```python
from build123d import *

# Parameters (mm, degrees)
SKETCH_W          = 28
SKETCH_H          = 22
PAD_DEPTH         = 52
FILLET_R          = 2
FILLET001_R       = 2
FILLET002_R       = 2
FILLET003_R       = 2
BOX_W             = 48
BOX_H             = 22.4
BOX_DEPTH         = 5.7
CYLINDER_R        = 1.5
CYLINDER_DEPTH    = 6
CYLINDER001_R     = 1.5
CYLINDER001_DEPTH = 6


with BuildPart() as part:
    # Sketch → Pad (new body)
    with BuildSketch(Plane.XZ):
        Rectangle(SKETCH_W, SKETCH_H)
    extrude(amount=PAD_DEPTH)

    # Fillet
    fillet_edges = [part.edges().sort_by_distance(p)[0] for p in [
        (-14, -26, 11),
    ]]
    fillet(fillet_edges, radius=FILLET_R)

    # Fillet001
    fillet001_edges = [part.edges().sort_by_distance(p)[0] for p in [
        (-14, -26, -11),
    ]]
    fillet(fillet001_edges, radius=FILLET001_R)

    # Fillet002
    fillet002_edges = [part.edges().sort_by_distance(p)[0] for p in [
        (14, -26, 11),
    ]]
    fillet(fillet002_edges, radius=FILLET002_R)

    # Fillet003
    fillet003_edges = [part.edges().sort_by_distance(p)[0] for p in [
        (14, -26, -11),
    ]]
    fillet(fillet003_edges, radius=FILLET003_R)

    # Box → Box (join)
    with BuildSketch(Plane(origin=(-24, 5.7, -11.2), x_dir=(1, 0, 0), z_dir=(0, -1, 0))):
        with Locations((24, 11.2)):
            Rectangle(BOX_W, BOX_H)
    extrude(amount=BOX_DEPTH)

    # Cylinder → Cylinder (join)
    with BuildSketch(Plane(origin=(-20, 0, 0), x_dir=(1, 0, 0), z_dir=(0, -1, 0))):
        Circle(CYLINDER_R)
    extrude(amount=CYLINDER_DEPTH)

    # Cylinder001 → Cylinder001 (join)
    with BuildSketch(Plane(origin=(20, 0, 0), x_dir=(1, 0, 0), z_dir=(0, -1, 0))):
        Circle(CYLINDER001_R)
    extrude(amount=CYLINDER001_DEPTH)


solid = part.part
```
Model file for the job. Use its own axes, mm. A direction names the side the tool comes from. Coordinates: 2 decimals unless noted, no trailing zeros. Loops run counter-clockwise (first coordinate to the right, second up) from the corner with the lowest first, then second, coordinate; pieces in that order, holes last. Notation, with made-up numbers: (26, 61.25) - (45, 61.25) arc R22 ccw to (45, 76.25) - close; hole circle Ø9 at (53, 41.25). An arc over 180 degrees is marked (long way). Answer as a JSON object with one key per item and string values. Group by question number.
(1) Two-plate mould, pull along X, no slides. Class faces 1 (the face through (-21.5, -2.96, 0.07)), 2 (the face through (18.5, -2.96, 0.07)), 3 (the face through (13.43, -26.36, -10.4)), 4 (the face through (0, 3, -11.2)): released by +X, released by -X, zero draft, split by the parting line, or undercut.
(2) Probe line 1 along X through (y, z) = (-22, 8.5); line 2 along Z through (x, y) = (-0.5, -37); line 3 along Y through (x, z) = (-16, -3.25). List the from-to ranges inside material, lowest first.
(3) Cut at D-D (z = 0). Give the cut face in (x, y), then the cut area to 3 significant figures.
(4) Cut at C-C (z = 6). Give the cut face in (x, y), then the cut area to 3 significant figures.
(5) Cut at A-A (y = -3). Give the cut face in (x, z).
(6) Tool access for faces 5 (the face through (-20, -6, 0)), 6 (the face through (0, -26, 11)), 7 (the face through (20, -6, 0)), 8 (the face through (-13.43, -26.36, -10.4)), 9 (the face through (13.4, -26.36, 10.43)): list every direction of +Z, -Z, +X, -X, +Y, -Y with a clear straight run to the whole face (end or side of a thin tool).
(7) Flat gauge pins, fed straight in: pin 1 (1 mm diameter, centred on y = -10.5, z = -2, fed in from -X); pin 2 (6 mm diameter, centred on y = -25.5, z = -8, fed in from +X); pin 3 (19 mm diameter, centred on x = 0, y = -33, fed in from -Z). Where does each tip first touch, or does it go through?
(8) Cut at B-B (x = -3). Give the cut face in (y, z).
Geometry says:
{
 "1": {"face 1": "undercut", "face 2": "undercut", "face 3": "released by +X", "face 4": "zero draft"},
 "2": {"line 1": "x = -14 to 14", "line 2": "z = -11 to 11", "line 3": "y = 0 to 5.7"},
 "3": {"outline": "(-24, 0) - (-21.5, 0) - (-21.5, -6) - (-18.5, -6) - (-18.5, 0) - (-14, 0) - (-14, -52) - (14, -52) - (14, 0) - (18.5, 0) - (18.5, -6) - (21.5, -6) - (21.5, 0) - (24, 0) - (24, 5.7) - (-24, 5.7) - close", "area": "1,770 mm^2"},
 "4": {"outline": "(-24, 0) - (-14, 0) - (-14, -52) - (14, -52) - (14, 0) - (24, 0) - (24, 5.7) - (-24, 5.7) - close", "area": "1,730 mm^2"},
 "5": {"outline": "circle Ø3 at (-20, 0); (-14, -9) arc R2 ccw to (-12, -11) - (12, -11) arc R2 ccw to (14, -9) - (14, 9) arc R2 ccw to (12, 11) - (-12, 11) arc R2 ccw to (-14, 9) - close; circle Ø3 at (20, 0)"},
 "6": {"face 5": "+Z, -Z, -X, -Y", "face 6": "+Z, +X, -X, -Y", "face 7": "+Z, -Z, +X, -Y", "face 8": "-Z, -X, -Y", "face 9": "+Z, +X, -Y"},
 "7": {"pin 1": "stops at x = -14", "pin 2": "stops at x = 14", "pin 3": "stops at z = -11"},
 "8": {"outline": "(-52, -11) - (0, -11) - (0, -11.2) - (5.7, -11.2) - (5.7, 11.2) - (0, 11.2) - (0, 11) - (-52, 11) - close"}
}
